For this review, take the finished solid that the model builds, in its own axes (mm). A direction names the side the tool comes from. Give positions to 0.01 mm unless a question says otherwise; leave off trailing zeros. Write each loop counter-clockwise with the first axis right and the second up, starting at its lowest first coordinate (ties: lowest second). Pieces come first, ordered by that corner, then holes. Notation, with made-up numbers: M -27.5,64 L 17.5,64 A37 ccw 17.5,101 Z; hole C 0.25,21 d2. An arc over 180 degrees is marked long. Answer as a JSON object with one key per item and string values. Group by question number.
```python
from build123d import *

# Parameters (mm, degrees)
BOSS_EXTRUDE1_DEPTH = 4.7625
CUT_EXTRUDE1_REACH  = 129.016
SKETCH3_R           = 10.16
SKETCH3_R_2         = 3.556
SKETCH3_R_3         = 1.75
SKETCH3_R_4         = 3.4925
SKETCH3_R_5         = 4.064
SKETCH3_W           = 71.35
SKETCH3_H           = 24.35
SKETCH4_W           = 6.35
SKETCH4_H           = 21
BOSS_EXTRUDE2_DEPTH = 19.05
SKETCH5_R           = 2.25
CUT_EXTRUDE2_DEPTH  = 212.413611199
BOSS_EXTRUDE3_DEPTH = 2.54
BOSS_EXTRUDE4_DEPTH = 2.54
FILLET1_R           = 6.35


with BuildPart() as part:
    # Sketch2 → Boss-Extrude1 (new body)
    with BuildSketch(Plane(origin=(0, 0, 0), x_dir=(1, 0, 0), z_dir=(0, 1, 0))):
        Polygon((-109.9, 0), (109.9, 0), (109.9, -63.5), (84.5, -63.5), (84.5, -42.5), (63.5, -42.5), (63.5, -63.5), (-63.5, -63.5), (-63.5, -42.5), (-84.5, -42.5), (-84.5, -63.5), (-109.9, -63.5), align=None)
    extrude(amount=BOSS_EXTRUDE1_DEPTH)

    # Sketch3 → Cut-Extrude1 (cut, up to next)
    with BuildSketch(Plane(origin=(0, 4.7625, 0), x_dir=(1, 0, 0), z_dir=(0, 1, 0)), mode=Mode.PRIVATE) as cut_extrude1_sk1:
        with Locations(Location((-84.5, -21.25, 0), (0, 0, 270))):
            Circle(SKETCH3_R)
    cut_extrude1_tool1 = extrude(cut_extrude1_sk1.sketch, amount=-CUT_EXTRUDE1_REACH, mode=Mode.PRIVATE) & part.part
    # Sketch3 → Cut-Extrude1 (cut, up to next)
    with BuildSketch(Plane(origin=(0, 4.7625, 0), x_dir=(1, 0, 0), z_dir=(0, 1, 0)), mode=Mode.PRIVATE) as cut_extrude1_sk2:
        with Locations(Location((-59.1, -21.25, 0), (0, 0, 270))):
            Circle(SKETCH3_R_2)
    cut_extrude1_tool2 = extrude(cut_extrude1_sk2.sketch, amount=-CUT_EXTRUDE1_REACH, mode=Mode.PRIVATE) & part.part
    # Sketch3 → Cut-Extrude1 (cut, up to next)
    with BuildSketch(Plane(origin=(0, 4.7625, 0), x_dir=(1, 0, 0), z_dir=(0, 1, 0)), mode=Mode.PRIVATE) as cut_extrude1_sk3:
        with Locations(Location((-37.5, -38.5, 0), (0, 0, 270))):
            Circle(SKETCH3_R_3)
    cut_extrude1_tool3 = extrude(cut_extrude1_sk3.sketch, amount=-CUT_EXTRUDE1_REACH, mode=Mode.PRIVATE) & part.part
    # Sketch3 → Cut-Extrude1 (cut, up to next)
    with BuildSketch(Plane(origin=(0, 4.7625, 0), x_dir=(1, 0, 0), z_dir=(0, 1, 0)), mode=Mode.PRIVATE) as cut_extrude1_sk4:
        with Locations(Location((-37.5, -7.5, 0), (0, 0, 270))):
            Circle(SKETCH3_R_3)
    cut_extrude1_tool4 = extrude(cut_extrude1_sk4.sketch, amount=-CUT_EXTRUDE1_REACH, mode=Mode.PRIVATE) & part.part
    # Sketch3 → Cut-Extrude1 (cut, up to next)
    with BuildSketch(Plane(origin=(0, 4.7625, 0), x_dir=(1, 0, 0), z_dir=(0, 1, 0)), mode=Mode.PRIVATE) as cut_extrude1_sk5:
        with Locations(Location((37.5, -38.5, 0), (0, 0, 90))):
            Circle(SKETCH3_R_3)
    cut_extrude1_tool5 = extrude(cut_extrude1_sk5.sketch, amount=-CUT_EXTRUDE1_REACH, mode=Mode.PRIVATE) & part.part
    # Sketch3 → Cut-Extrude1 (cut, up to next)
    with BuildSketch(Plane(origin=(0, 4.7625, 0), x_dir=(1, 0, 0), z_dir=(0, 1, 0)), mode=Mode.PRIVATE) as cut_extrude1_sk6:
        with Locations(Location((37.5, -7.5, 0), (0, 0, 90))):
            Circle(SKETCH3_R_3)
    cut_extrude1_tool6 = extrude(cut_extrude1_sk6.sketch, amount=-CUT_EXTRUDE1_REACH, mode=Mode.PRIVATE) & part.part
    # Sketch3 → Cut-Extrude1 (cut, up to next)
    with BuildSketch(Plane(origin=(0, 4.7625, 0), x_dir=(1, 0, 0), z_dir=(0, 1, 0)), mode=Mode.PRIVATE) as cut_extrude1_sk7:
        with Locations(Location((54.725, -23, 0), (0, 0, 270))):
            Circle(SKETCH3_R_4)
    cut_extrude1_tool7 = extrude(cut_extrude1_sk7.sketch, amount=-CUT_EXTRUDE1_REACH, mode=Mode.PRIVATE) & part.part
    # Sketch3 → Cut-Extrude1 (cut, up to next)
    with BuildSketch(Plane(origin=(0, 4.7625, 0), x_dir=(1, 0, 0), z_dir=(0, 1, 0)), mode=Mode.PRIVATE) as cut_extrude1_sk8:
        with Locations(Location((84.5, -23, 0), (0, 0, 270))):
            Circle(SKETCH3_R_5)
    cut_extrude1_tool8 = extrude(cut_extrude1_sk8.sketch, amount=-CUT_EXTRUDE1_REACH, mode=Mode.PRIVATE) & part.part
    # Sketch3 → Cut-Extrude1 (cut, up to next)
    with BuildSketch(Plane(origin=(0, 4.7625, 0), x_dir=(1, 0, 0), z_dir=(0, 1, 0)), mode=Mode.PRIVATE) as cut_extrude1_sk9:
        with Locations((0, -23)):
            Rectangle(SKETCH3_W, SKETCH3_H)
    cut_extrude1_tool9 = extrude(cut_extrude1_sk9.sketch, amount=-CUT_EXTRUDE1_REACH, mode=Mode.PRIVATE) & part.part
    add(cut_extrude1_tool1.solids().sort_by_distance((-84.5, 4.7625, 21.25))[0], mode=Mode.SUBTRACT)
    add(cut_extrude1_tool2.solids().sort_by_distance((-59.1, 4.7625, 21.25))[0], mode=Mode.SUBTRACT)
    add(cut_extrude1_tool3.solids().sort_by_distance((-37.5, 4.7625, 38.5))[0], mode=Mode.SUBTRACT)
    add(cut_extrude1_tool4.solids().sort_by_distance((-37.5, 4.7625, 7.5))[0], mode=Mode.SUBTRACT)
    add(cut_extrude1_tool5.solids().sort_by_distance((37.5, 4.7625, 38.5))[0], mode=Mode.SUBTRACT)
    add(cut_extrude1_tool6.solids().sort_by_distance((37.5, 4.7625, 7.5))[0], mode=Mode.SUBTRACT)
    add(cut_extrude1_tool7.solids().sort_by_distance((54.725, 4.7625, 23))[0], mode=Mode.SUBTRACT)
    add(cut_extrude1_tool8.solids().sort_by_distance((84.5, 4.7625, 23))[0], mode=Mode.SUBTRACT)
    add(cut_extrude1_tool9.solids().sort_by_distance((0, 4.7625, 23))[0], mode=Mode.SUBTRACT)

    # Sketch4 → Boss-Extrude2 (add)
    with BuildSketch(Plane.XZ):
        with Locations((-87.675, 53)):
            Rectangle(SKETCH4_W, SKETCH4_H)
        with Locations((87.675, 53)):
            Rectangle(SKETCH4_W, SKETCH4_H)
        with Locations((-60.325, 53)):
            Rectangle(SKETCH4_W, SKETCH4_H)
        with Locations((60.325, 53)):
            Rectangle(SKETCH4_W, SKETCH4_H)
    extrude(amount=BOSS_EXTRUDE2_DEPTH)

    # Sketch5 → Cut-Extrude2 (cut, through all)
    with BuildSketch(Plane(origin=(90.85, 0, 0), x_dir=(0, 0, -1), z_dir=(1, 0, 0))):
        with Locations((-53, -9.525)):
            Circle(SKETCH5_R)
    extrude(amount=-CUT_EXTRUDE2_DEPTH, mode=Mode.SUBTRACT)

    # Sketch6 → Boss-Extrude3 (add)
    with BuildSketch(Plane.XY.offset(63.5)):
        Polygon((90.85, -19.05), (109.9, 0), (90.85, 0), align=None)
        Polygon((57.15, -19.05), (38.1, 0), (57.15, 0), align=None)
        Polygon((-90.85, -19.05), (-90.85, 0), (-109.9, 0), align=None)
        Polygon((-57.15, -19.05), (-57.15, 0), (-38.1, 0), align=None)
    extrude(amount=-BOSS_EXTRUDE3_DEPTH)

    # Sketch7 → Boss-Extrude4 (add)
    with BuildSketch(Plane(origin=(0, 0, 42.5), x_dir=(-1, 0, 0), z_dir=(0, 0, -1))):
        Polygon((-90.85, -19.05), (-90.85, 0), (-109.9, 0), align=None)
        Polygon((-57.15, 0), (-38.1, 0), (-57.15, -19.05), align=None)
        Polygon((57.15, 0), (57.15, -19.05), (38.1, 0), align=None)
        Polygon((90.85, 0), (90.85, -19.05), (109.9, 0), align=None)
    extrude(amount=-BOSS_EXTRUDE4_DEPTH)

    # Fillet1
    # the kernel refuses this fillet: 6.35 mm, written as the material it takes off along each edge
    with BuildSketch(Plane(origin=(-79.375, -19.05, 42.5), x_dir=(0, 1, 0), z_dir=(1, 0, 0)), Plane(origin=(-41.275, -19.05, 63.5), x_dir=(0, 1, 0), z_dir=(-1, 0, 0)), Plane(origin=(79.375, -19.05, 42.5), x_dir=(0, 0, 1), z_dir=(-1, 0, 0)), Plane(origin=(68.625, -19.05, 42.5), x_dir=(0, 1, 0), z_dir=(1, 0, 0))) as fillet1_piece_1:
        with BuildLine():
            CenterArc((FILLET1_R, FILLET1_R), FILLET1_R, 180, 90)
            Line((0, FILLET1_R), (0, 0))
            Line((0, 0), (FILLET1_R, 0))
        make_face()
    extrude(amount=38.1, mode=Mode.SUBTRACT)
    with BuildSketch(Plane(origin=(41.275, -19.05, 63.5), x_dir=(0, 1, 0), z_dir=(1, 0, 0)), Plane(origin=(-68.625, -19.05, 63.5), x_dir=(0, 0, -1), z_dir=(-1, 0, 0)), Plane(origin=(-106.725, -19.05, 42.5), x_dir=(0, 0, 1), z_dir=(1, 0, 0)), Plane(origin=(106.725, -19.05, 63.5), x_dir=(0, 0, -1), z_dir=(-1, 0, 0))) as fillet1_piece_2:
        with BuildLine():
            CenterArc((FILLET1_R, -FILLET1_R), FILLET1_R, 90, 90)
            Line((0, -FILLET1_R), (0, 0))
            Line((0, 0), (FILLET1_R, 0))
        make_face()
    extrude(amount=38.1, mode=Mode.SUBTRACT)
    with BuildSketch(Plane(origin=(109.9, -15.875, 63.5), x_dir=(-1, 0, 0), z_dir=(0, 1, 0)), Plane(origin=(-109.9, -15.875, 0), x_dir=(1, 0, 0), z_dir=(0, 1, 0))) as fillet1_piece_3:
        with BuildLine():
            CenterArc((FILLET1_R, -FILLET1_R), FILLET1_R, 90, 90)
            Line((0, -FILLET1_R), (0, 0))
            Line((0, 0), (FILLET1_R, 0))
        make_face()
    extrude(amount=36.5125, mode=Mode.SUBTRACT)
    with BuildSketch(Plane(origin=(-109.9, -15.875, 63.5), x_dir=(1, 0, 0), z_dir=(0, 1, 0)), Plane(origin=(109.9, -15.875, 0), x_dir=(-1, 0, 0), z_dir=(0, 1, 0))) as fillet1_piece_4:
        with BuildLine():
            CenterArc((FILLET1_R, FILLET1_R), FILLET1_R, 180, 90)
            Line((0, FILLET1_R), (0, 0))
            Line((0, 0), (FILLET1_R, 0))
        make_face()
    extrude(amount=36.5125, mode=Mode.SUBTRACT)


solid = part.part
```
Item 1: Draft analysis for pull direction Z (two halves, no side actions). For faces 6 (the flat face through (-54, -6, 42.5)), 7 (the cylindrical face through (-62.255, 2.415, 22.891)), 8 (the flat face through (-74, 2, 42.5)), 9 (the flat face through (0, 2, 10.825)), state which applies: released by +Z, released by -Z, zero draft, split by the parting line, or undercut.
Item 2: Consider section A-A (x = -3.5). Give the boundary of the cut face in (y, z) (1 decimal).
Item 3: Machinability: for faces 1 (the flat face through (95, -6, 42.5)), 2 (the flat face through (-100, 0, 53)), 3 (the flat face through (98, -7, 60.96)), 4 (the flat face through (63.5, -5, 53)), 5 (the flat face through (-35.675, 2, 23)), which of the approach directions +Z, -Z, +X, -X, +Y, -Y give a long, thin tool a straight path to every point of the face, cutting with its end or side? Answer none if there is none.
Item 4: To check wall thickness, follow probe 1 along X at (y, z) = (-4.5, 53); probe 2 along Z at (x, y) = (37.5, 3.6); probe 3 along X at (y, z) = (1.1, 23) (1 decimal). State the ranges of each line that lie inside material, in increasing order.
Item 5: Insertion check: P1, Ø10, axis at x = 65, y = -15, coming from the -Z side; P2, Ø9.5, axis at x = 84.5, z = 23, coming from the -Y side; P3, Ø1.4, axis at x = -5.5, y = 2.5, coming from the -Z side; P4, Ø18.5, axis at x = -84.5, z = 21.25, coming from the -Y side. Each pin has a flat end and moves straight along its axis. Give the tip position at first contact, or say it passes through.
Item 6: Consider section B-B (z = 53). State how many separate pieces and enclosed holes the cut face has, plus the area to 3 significant figures.
Item 7: Consider section D-D (x = -48.5). Give the boundary of the cut face in (y, z), plus the area to 3 significant figures.
Result set:
{
 "1": {"face 6": "released by -Z", "face 7": "undercut", "face 8": "released by +Z", "face 9": "undercut"},
 "2": {"outline": "M 0,0 L 4.8,0 L 4.8,10.8 L 0,10.8 Z; M 0,35.2 L 4.8,35.2 L 4.8,63.5 L 0,63.5 Z"},
 "3": {"face 1": "-Z, +X, -X, -Y", "face 2": "-X, -Y", "face 3": "+X, -Y", "face 4": "+Z, +Y, -Y", "face 5": "+Y, -Y"},
 "4": {"probe 1": "x = -90.85 to -84.5, -63.5 to -57.15, 57.15 to 63.5, 84.5 to 90.85", "probe 2": "z = 0 to 5.75, 9.25 to 36.75, 40.25 to 63.5", "probe 3": "x = -109.9 to -94.5, -74.5 to -62.2, -56 to -35.7, 35.7 to 51.2, 58.2 to 80.4, 88.6 to 109.9"},
 "5": {"P1": "stops at z = 42.5", "P2": "stops at y = 0", "P3": "stops at z = 0", "P4": "passes through"},
 "6": {"separate pieces": "7", "enclosed holes": "0", "area": "1,220 mm^2"},
 "7": {"outline": "M -10.4,42.5 L 0,42.5 L 0,0 L 4.76,0 L 4.76,63.5 L -10.4,63.5 L -10.4,60.96 L 0,60.96 L 0,45.04 L -10.4,45.04 Z", "area": "355 mm^2"}
}
